Check sheet for the drawn part. Datum: minimum x, y, z corner. Units: mm. A direction names the side the tool comes from. Coordinates: 2 decimals unless noted, no trailing zeros. Write each loop counter-clockwise with the first axis right and the second up, starting at its lowest first coordinate (ties: lowest second). Pieces come first, ordered by that corner, then holes. Notation, with made-up numbers: (72, -16) -> (76, -16) arc R23 cw to (76, 1) -> close; hole circle Ø1 at (42, 52). An arc over 180 degrees is marked (long way). One line per question, with ' | ' between items.
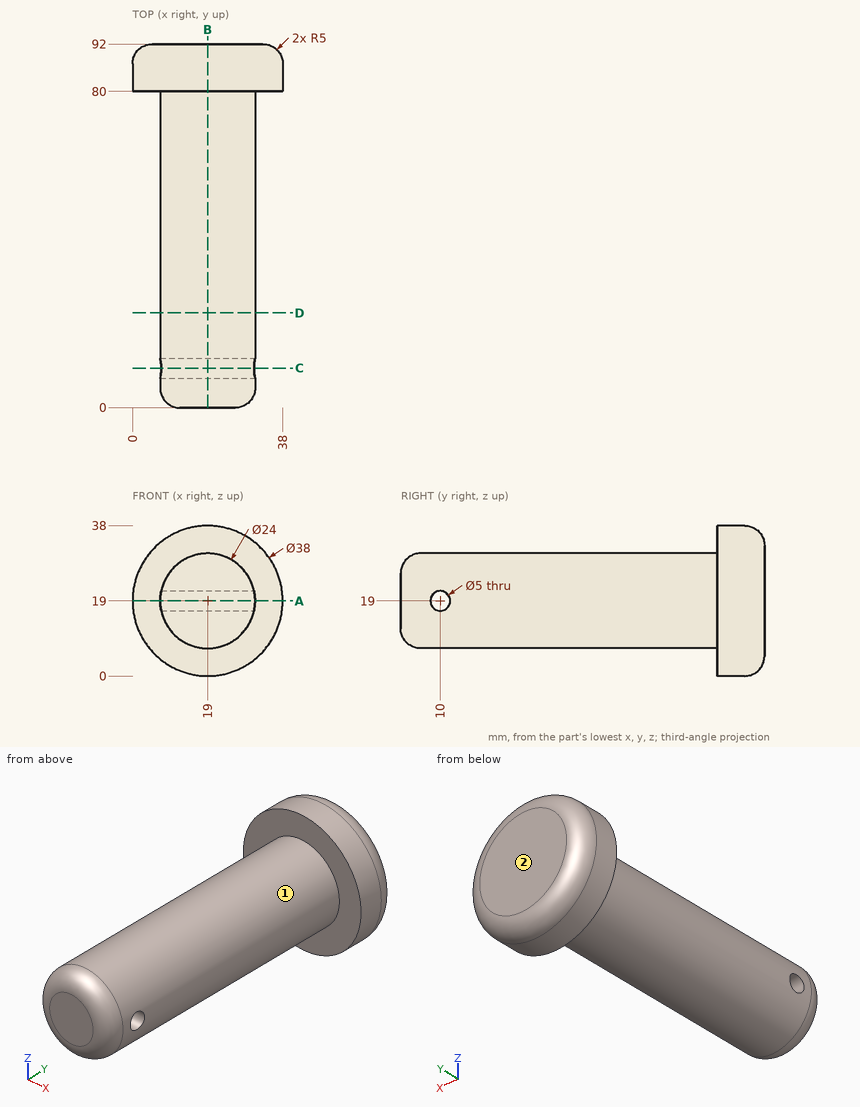
1. Cross-section at D-D on y = 24. Record the boundary of the cut face in (x, z).
Worked answers:
outline: circle Ø24 at (19, 19)
2. Tool access check on the marked faces 1 and 2. Record the directions out of +Z, -Z, +X, -X, +Y, -Y that give a thin tool (end or side, any length) a straight path to the whole face; none if there is none.
Worked answers:
face 1: -Y | face 2: +Z, -Z, +X, -X, +Y
3. Material ranges on line 1 (Y direction, x = 22.75, z = 19); line 2 (Y direction, x = 8, z = 24); line 3 (X direction, y = 65.5, z = 18.5), recorded low to high. Write a range as from..to.
Worked answers:
line 1: 0..7.5, 12.5..92 | line 2: 80..92 | line 3: 7.01..30.99
4. Cross-section at A-A on z = 19. Record the boundary of the cut face in (x, y).
Worked answers:
outline: (0, 80) -> (7, 80) -> (7, 12.5) -> (31, 12.5) -> (31, 80) -> (38, 80) -> (38, 87) arc R5 ccw to (33, 92) -> (5, 92) arc R5 ccw to (0, 87) -> close; (7, 5) arc R5 ccw to (12, 0) -> (26, 0) arc R5 ccw to (31, 5) -> (31, 7.5) -> (7, 7.5) -> close
5. Go/stop test with flat-tipped pins: P1, Ø6, axis at y = 81.5, z = 15, coming from the -X side; P2, Ø3, axis at x = 13, y = 82, coming from the +Z side; P3, Ø4, axis at y = 16, z = 14, coming from the +X side; P4, Ø4, axis at y = 38.5, z = 33.5, coming from the -X side. Record where each tip stops, or that it passes through.
Worked answers:
P1: x = 0.03 | P2: z = 37.46 | P3: x = 30.62 | P4: through
6. Cross-section at B-B on x = 19. Record the boundary of the cut face in (y, z).
Worked answers:
outline: (0, 12) arc R5 ccw to (5, 7) -> (80, 7) -> (80, 0) -> (87, 0) arc R5 ccw to (92, 5) -> (92, 33) arc R5 ccw to (87, 38) -> (80, 38) -> (80, 31) -> (5, 31) arc R5 ccw to (0, 26) -> close; hole circle Ø5 at (10, 19)
7. Cross-section at C-C on y = 10. Record the boundary of the cut face in (x, z).
Worked answers:
outline: (7.26, 16.5) arc R12 ccw to (30.74, 16.5) -> close; (7.26, 21.5) -> (30.74, 21.5) arc R12 ccw to start
